Source: CAD feature listing. Evaluate the final solid. Frame: model axes, mm. Round coordinates to 2 decimals unless told otherwise and drop trailing zeros. Order: outer loops, then holes, each group sorted by start corner. A loop starts at its lowest first (then second) coordinate and runs counter-clockwise, first axis right, second up. Notation, with made-up numbers: M 38.25,-5 L 74.25,-5 A29 ccw 74.25,30 Z; hole C 22,4 d8. An arc over 180 degrees is marked long. Answer as CSV lines item,"result". Start each with the question number.
Item 1: Section query A-A on y = 1534. Return the cut outline in (x, z), plus the area to 3 significant figures.
Item 2: Line query: line 1 (X direction, y = 1201, z = 4.5); line 2 (Z direction, x = 18.75, y = 1925). Output: solid intervals per line, ascending. Write a range as [from, to].
Item 3: First-contact query: P1, Ø15, axis at x = -2.5, y = 782.5, coming from the -Z side; P2, Ø1.5, axis at y = 1507, z = -16, coming from the +X side; P3, Ø10.5, axis at x = 0, y = 1880, coming from the +Z side; P4, Ø7, axis at y = 800, z = 0, coming from the +X side. Flat tips, straight axial feed; report the tip coordinate or a pass-through.
Autodesk Inventor part; units mm, degrees
ref_plane "YZ Plane" through (0, 0, 0) normal (1, 0, 0) x (0, 1, 0)
ref_plane "XZ Plane" through (0, 0, 0) normal (0, 1, 0) x (-1, 0, 0)
ref_plane "XY Plane" through (0, 0, 0) normal (0, 0, 1) x (1, 0, 0)
sketch "Sketch1" plane through (0, 0, 0) normal (0, 1, 0) x (-1, 0, 0)
  line L0 (15, 20) -> (-15, 20)
  line L1 (-20, 15) -> (-20, -15)
  line L2 (-15, -20) -> (15, -20)
  line L3 (20, -15) -> (20, 15)
  line L4 (20, 20) -> (-20, -20) construction
  line L5 (-20, 20) -> (20, -20) construction
  line L6 (13, 18) -> (-13, 18)
  line L7 (-18, 13) -> (-18, -13)
  line L8 (-13, -18) -> (13, -18)
  line L9 (18, -13) -> (18, 13)
  line L10 (18, 18) -> (-18, -18) construction
  line L11 (-18, 18) -> (18, -18) construction
  line L12 (35, 35) -> (-35, 35)
  line L13 (-35, 35) -> (-35, -35)
  line L14 (-35, -35) -> (35, -35)
  line L15 (35, -35) -> (35, 35)
  line L16 (35, 35) -> (-35, -35) construction
  line L17 (-35, 35) -> (35, -35) construction
  arc A0 (20, 15) -> (15, 20) centre (15, 15) ccw
  arc A1 (18, 13) -> (13, 18) centre (13, 13) ccw
  arc A2 (13, -18) -> (18, -13) centre (13, -13) ccw
  arc A3 (15, -20) -> (20, -15) centre (15, -15) ccw
  arc A4 (-13, 18) -> (-18, 13) centre (-13, 13) ccw
  arc A5 (-15, 20) -> (-20, 15) centre (-15, 15) ccw
  arc A6 (-20, -15) -> (-15, -20) centre (-15, -15) ccw
  arc A7 (-18, -13) -> (-13, -18) centre (-13, -13) ccw
  point P0 (0, 0)
  dimension "d0" = 40
  dimension "d1" = 40
  dimension "d2" = 36
  dimension "d3" = 36
  dimension "d4" = 70
  dimension "d5" = 70
  dimension "d6" = 5
extrude "Extrusion1" add sketch "Sketch1" along normal blind 3 contours L15 L14 L13 L12
extrude "Extrusion2" add sketch "Sketch1" along normal blind 2000 contours A0 L3 A3 L2 A6 L1 A5 L0
sketch "Sketch2" plane through (20, 3, -15) normal (1, 0, 0) x (0, 0, -1)
  line L0 (-30, 0) -> (-30, 1997)
  line L1 (-30, 1997) -> (0, 1997)
  point P0 (-15, -3)
  point P1 (-15, 1197)
  point P2 (-15, 1147)
  dimension "d18" = 50
  dimension "d19" = 15
  dimension "d20" = 15
  dimension "d21" = 800
hole "Hole1" at (20, 1200, 0) at (20, 1150, 0) direction (-1, 0, 0) diameter 8 end through all
sketch "Sketch3" plane through (15, 3, 20) normal (0, 0, 1) x (1, 0, 0)
  line L0 (-30, 0) -> (-30, 1997)
  line L1 (-30, 1997) -> (0, 1997)
  point P0 (-15, -3)
  point P1 (-15, 1197)
  point P2 (-15, 1147)
  dimension "d29" = 50
  dimension "d30" = 15
  dimension "d31" = 15
  dimension "d32" = 800
hole "Hole2" at (0, 1200, 20) at (0, 1150, 20) direction (0, 0, -1) diameter 8 end through all
sketch "Sketch4" plane through (20, 3, -15) normal (1, 0, 0) x (0, 0, -1)
  line L0 (-30, 0) -> (-30, 1997)
  line L1 (0, 0) -> (-30, 0)
  point P0 (-15, -3)
  point P1 (-15, 150)
  point P2 (-15, 100)
  dimension "d40" = 50
  dimension "d41" = 15
  dimension "d42" = 15
  dimension "d43" = 100
hole "Hole3" at (20, 153, 0) at (20, 103, 0) direction (-1, 0, 0) diameter 8 end through all
sketch "Sketch5" plane through (15, 3, 20) normal (0, 0, 1) x (1, 0, 0)
  line L0 (0, 0) -> (0, 1997)
  line L1 (0, 0) -> (-30, 0)
  point P0 (-15, -3)
  point P1 (-15, 150)
  point P2 (-15, 100)
  dimension "d51" = 50
  dimension "d52" = 15
  dimension "d53" = 15
  dimension "d54" = 100
hole "Hole4" at (0, 153, 20) at (0, 103, 20) direction (0, 0, -1) diameter 8 end through all
sketch "Sketch6" plane through (15, 3, 20) normal (0, 0, 1) x (1, 0, 0)
  line L0 (-30, 1997) -> (0, 1997)
  line L1 (-30, 0) -> (-30, 1997)
  point P0 (-15, -3)
  point P1 (-15, 1972)
  point P2 (-15, 1922)
  dimension "d62" = 50
  dimension "d63" = 25
  dimension "d64" = 15
  dimension "d65" = 15
hole "Hole5" at (0, 1975, 20) at (0, 1925, 20) direction (0, 0, -1) diameter 8 end through all
sketch "Sketch7" plane through (20, 3, -15) normal (1, 0, 0) x (0, 0, -1)
  line L0 (-30, 1997) -> (0, 1997)
  line L1 (-30, 0) -> (-30, 1997)
  point P0 (-15, -3)
  point P1 (-15, 1972)
  point P2 (-15, 1922)
  dimension "d73" = 25
  dimension "d74" = 50
  dimension "d75" = 15
  dimension "d76" = 15
hole "Hole6" at (20, 1975, 0) at (20, 1925, 0) direction (-1, 0, 0) diameter 8 end through all
sketch "Sketch9" plane through (20, 3, -15) normal (1, 0, 0) x (0, 0, -1)
  line L0 (0, 0) -> (0, 1997)
  circle A0 centre (-15, 1147) radius 4
  point P0 (-15, -3)
  point P1 (-15, 847)
  point P2 (-15, 797)
  dimension "d95" = 50
  dimension "d96" = 15
  dimension "d97" = 15
  dimension "d98" = 300
hole "Hole8" at (20, 850, 0) at (20, 800, 0) direction (-1, 0, 0) diameter 8 end through all
sketch "Sketch10" plane through (15, 3, 20) normal (0, 0, 1) x (1, 0, 0)
  line L0 (0, 0) -> (0, 1997)
  circle A0 centre (-15, 1147) radius 4
  point P0 (-15, -3)
  point P1 (-15, 847)
  point P2 (-15, 797)
  dimension "d106" = 50
  dimension "d107" = 15
  dimension "d108" = 15
  dimension "d109" = 300
hole "Hole9" at (0, 850, 20) at (0, 800, 20) direction (0, 0, -1) diameter 8 end through all
sketch "Sketch11" plane through (15, 3, 20) normal (0, 0, 1) x (1, 0, 0)
  line L0 (0, 0) -> (0, 1997)
  line L1 (-30, 1997) -> (0, 1997)
  point P0 (-15, -3)
  point P1 (-15, 1877)
  point P2 (-15, 1827)
  dimension "d117" = 50
  dimension "d118" = 15
  dimension "d119" = 15
  dimension "d120" = 120
hole "Hole10" at (0, 1880, 20) at (0, 1830, 20) direction (0, 0, -1) diameter 8 end through all
sketch "Sketch12" plane through (20, 3, -15) normal (1, 0, 0) x (0, 0, -1)
  line L0 (0, 0) -> (0, 1997)
  line L1 (-30, 1997) -> (0, 1997)
  point P0 (-15, -3)
  point P1 (-15, 1877)
  point P2 (-15, 1827)
  dimension "d128" = 50
  dimension "d129" = 15
  dimension "d130" = 15
  dimension "d131" = 120
hole "Hole11" at (20, 1880, 0) at (20, 1830, 0) direction (-1, 0, 0) diameter 8 end through all
properties part number "metal supporter"
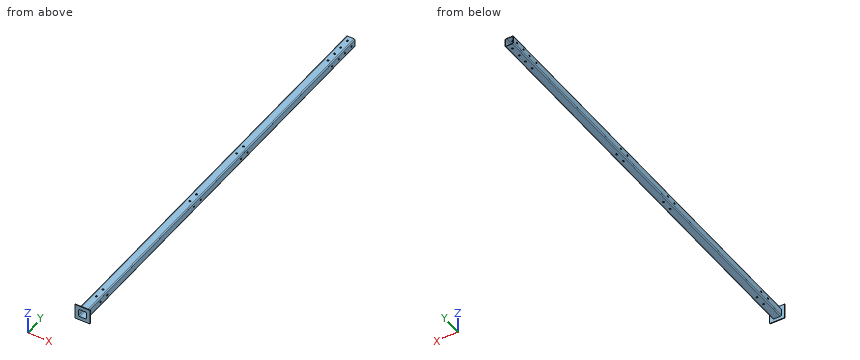
Results:
1,outline,"M -20,-15 A5 ccw -15,-20 L 15,-20 A5 ccw 20,-15 L 20,15 A5 ccw 15,20 L -15,20 A5 ccw -20,15 Z; hole M -18,-13 A5 ccw -13,-18 L 13,-18 A5 ccw 18,-13 L 18,13 A5 ccw 13,18 L -13,18 A5 ccw -18,13 Z"
1,area,"304 mm^2"
2,line 1,"[-20, -18], [18, 20]"
2,line 2,"[-18.31, -4], [4, 18.31]"
3,P1,"z = -20"
3,P2,"x = 19.99"
3,P3,"z = 20"
3,P4,"through"
